Work out the finished part from the listing and answer in its coordinate system (mm). A direction names the side the tool comes from. Round coordinates to 2 decimals unless told otherwise and drop trailing zeros. Order: outer loops, then holes, each group sorted by start corner. A loop starts at its lowest first (then second) coordinate and runs counter-clockwise, first axis right, second up. Notation, with made-up numbers: (33.25, 48) - (79.25, 48) arc R17 ccw to (79.25, 53) - close; hole circle Ø2 at (50, -11.75). An arc over 180 degrees is marked (long way). Use one line per item in the form item = value. Start each with the question number.
Q1. For a pull along Y with two mould halves and no side action, classify faces 1 (the flat face through (-1, 10.514, -12)), 2 (the flat face through (40.64, 38, -20)), 3 (the cylindrical face through (39.388, 64.993, -18.568)) as +Y half, -Y half, draft (parallel to the pull), parting line (faces both ways), or undercut.
Q2. The part is cut by section C-C on y = 25.5. Determine the outline of the cut face in (x, z).
Q3. Which of the six approach directions +Z, -Z, +X, -X, +Y, -Y give full straight-line access (tool end or side, diameter ignored) to faces 4 (the flat face through (0, 62, -11)), 5 (the flat face through (19, 38, -25.4)), 6 (the flat face through (-1, 11.594, -1))?
Q4. The part is cut by section B-B on z = -11.43. State how many separate pieces and enclosed holes the cut face has, plus the area to 3 significant figures.
Q5. Given P1, Ø2.5, axis at y = 6.64, z = -16.38, coming from the -X side; P2, Ø3.5, axis at y = 67.16, z = -19.05, coming from the +X side; P3, Ø4, axis at x = 36, z = -18.5, coming from the +Y side, each flat-ended and moving along its own axis, determine where each tip first touches the part or whether it passes through.
Q6. Find the intervals of material crossed by line 1 (Y direction, x = 39.3, z = -19.05); line 2 (Z direction, x = 29.5, y = 38.5); line 3 (X direction, y = 53, z = -21.25), in increasing order. Write a range as [from, to].
from build123d import *

# Parameters (mm, degrees)
SKETCH1_W           = 43.18
SKETCH1_H           = 27.94
SKETCH1_W_2         = 38.1
SKETCH1_H_2         = 22.86
BOSS_EXTRUDE1_DEPTH = 76.2
CUT_EXTRUDE1_REACH  = 93.193
SKETCH3_R           = 2.2225
SKETCH3_R_2         = 6.99999997
CUT_EXTRUDE2_REACH  = 93.193
SKETCH2_W           = 19.91868
SKETCH2_H           = 38.1
SKETCH2_W_2         = 1.47066
SKETCH2_H_2         = 1.0795
SKETCH2_R           = 2.2225
FILLET1_R           = 1.27
FILLET2_R           = 1.27


# Some blends are built 0.0001 mm under size
with BuildPart() as part:
    # Sketch1 → Boss-Extrude1 (new body)
    with BuildSketch(Plane(origin=(0, 0, 0), x_dir=(1, 0, 0), z_dir=(0, 1, 0))):
        with Locations((19.05, 11.43)):
            Rectangle(SKETCH1_W, SKETCH1_H)
        with Locations((19.05, 11.43)):
            Rectangle(SKETCH1_W_2, SKETCH1_H_2, mode=Mode.SUBTRACT)
    extrude(amount=BOSS_EXTRUDE1_DEPTH)

    # Sketch3 → Cut-Extrude1 (cut, up to next)
    with BuildSketch(Plane(origin=(40.64, 0, 0), x_dir=(0, 0, -1), z_dir=(1, 0, 0)), mode=Mode.PRIVATE) as cut_extrude1_sk1:
        with Locations((19.05, 67.16268)):
            Circle(SKETCH3_R)
    cut_extrude1_tool1 = extrude(cut_extrude1_sk1.sketch, amount=-CUT_EXTRUDE1_REACH, mode=Mode.PRIVATE) & part.part
    # Sketch3 → Cut-Extrude1 (cut, up to next)
    with BuildSketch(Plane(origin=(40.64, 0, 0), x_dir=(0, 0, -1), z_dir=(1, 0, 0)), mode=Mode.PRIVATE) as cut_extrude1_sk2:
        with Locations((3.81, 67.16268)):
            Circle(SKETCH3_R)
    cut_extrude1_tool2 = extrude(cut_extrude1_sk2.sketch, amount=-CUT_EXTRUDE1_REACH, mode=Mode.PRIVATE) & part.part
    # Sketch3 → Cut-Extrude1 (cut, up to next)
    with BuildSketch(Plane(origin=(40.64, 0, 0), x_dir=(0, 0, -1), z_dir=(1, 0, 0)), mode=Mode.PRIVATE) as cut_extrude1_sk3:
        with Locations((19.05, 13.82268)):
            Circle(SKETCH3_R)
    cut_extrude1_tool3 = extrude(cut_extrude1_sk3.sketch, amount=-CUT_EXTRUDE1_REACH, mode=Mode.PRIVATE) & part.part
    # Sketch3 → Cut-Extrude1 (cut, up to next)
    with BuildSketch(Plane(origin=(40.64, 0, 0), x_dir=(0, 0, -1), z_dir=(1, 0, 0)), mode=Mode.PRIVATE) as cut_extrude1_sk4:
        with Locations((3.81, 13.82268)):
            Circle(SKETCH3_R)
    cut_extrude1_tool4 = extrude(cut_extrude1_sk4.sketch, amount=-CUT_EXTRUDE1_REACH, mode=Mode.PRIVATE) & part.part
    # Sketch3 → Cut-Extrude1 (cut, up to next)
    with BuildSketch(Plane(origin=(40.64, 0, 0), x_dir=(0, 0, -1), z_dir=(1, 0, 0)), mode=Mode.PRIVATE) as cut_extrude1_sk5:
        with Locations((11.43, 40.49268)):
            Circle(SKETCH3_R_2)
    cut_extrude1_tool5 = extrude(cut_extrude1_sk5.sketch, amount=-CUT_EXTRUDE1_REACH, mode=Mode.PRIVATE) & part.part
    add(cut_extrude1_tool1.solids().sort_by_distance((40.64, 67.16268, -19.05))[0], mode=Mode.SUBTRACT)
    add(cut_extrude1_tool2.solids().sort_by_distance((40.64, 67.16268, -3.81))[0], mode=Mode.SUBTRACT)
    add(cut_extrude1_tool3.solids().sort_by_distance((40.64, 13.82268, -19.05))[0], mode=Mode.SUBTRACT)
    add(cut_extrude1_tool4.solids().sort_by_distance((40.64, 13.82268, -3.81))[0], mode=Mode.SUBTRACT)
    add(cut_extrude1_tool5.solids().sort_by_distance((40.64, 40.49268, -11.43))[0], mode=Mode.SUBTRACT)

    # Sketch2 → Cut-Extrude2 (cut, up to next)
    with BuildSketch(Plane.ZY.offset(2.54), mode=Mode.PRIVATE) as cut_extrude2_sk1:
        with Locations((-11.43, 30.64383099)):
            Rectangle(SKETCH2_W, SKETCH2_H)
    cut_extrude2_tool1 = extrude(cut_extrude2_sk1.sketch, amount=-CUT_EXTRUDE2_REACH, mode=Mode.PRIVATE) & part.part
    # Sketch2 → Cut-Extrude2 (cut, up to next)
    with BuildSketch(Plane.ZY.offset(2.54), mode=Mode.PRIVATE) as cut_extrude2_sk2:
        with Locations((-22.12467, 30.64383099)):
            Rectangle(SKETCH2_W_2, SKETCH2_H)
    cut_extrude2_tool2 = extrude(cut_extrude2_sk2.sketch, amount=-CUT_EXTRUDE2_REACH, mode=Mode.PRIVATE) & part.part
    # Sketch2 → Cut-Extrude2 (cut, up to next)
    with BuildSketch(Plane.ZY.offset(2.54), mode=Mode.PRIVATE) as cut_extrude2_sk3:
        with Locations((-11.43, 50.23358099)):
            Rectangle(SKETCH2_W, SKETCH2_H_2)
    cut_extrude2_tool3 = extrude(cut_extrude2_sk3.sketch, amount=-CUT_EXTRUDE2_REACH, mode=Mode.PRIVATE) & part.part
    # Sketch2 → Cut-Extrude2 (cut, up to next)
    with BuildSketch(Plane.ZY.offset(2.54), mode=Mode.PRIVATE) as cut_extrude2_sk4:
        with Locations((-0.73533, 30.64383099)):
            Rectangle(SKETCH2_W_2, SKETCH2_H)
    cut_extrude2_tool4 = extrude(cut_extrude2_sk4.sketch, amount=-CUT_EXTRUDE2_REACH, mode=Mode.PRIVATE) & part.part
    # Sketch2 → Cut-Extrude2 (cut, up to next)
    with BuildSketch(Plane.ZY.offset(2.54), mode=Mode.PRIVATE) as cut_extrude2_sk5:
        with Locations((-11.43, 11.05408099)):
            Rectangle(SKETCH2_W, SKETCH2_H_2)
    cut_extrude2_tool5 = extrude(cut_extrude2_sk5.sketch, amount=-CUT_EXTRUDE2_REACH, mode=Mode.PRIVATE) & part.part
    # Sketch2 → Cut-Extrude2 (cut, up to next)
    with BuildSketch(Plane.ZY.offset(2.54), mode=Mode.PRIVATE) as cut_extrude2_sk6:
        with Locations((-6.47954, 6.64337099)):
            Circle(SKETCH2_R)
    cut_extrude2_tool6 = extrude(cut_extrude2_sk6.sketch, amount=-CUT_EXTRUDE2_REACH, mode=Mode.PRIVATE) & part.part
    # Sketch2 → Cut-Extrude2 (cut, up to next)
    with BuildSketch(Plane.ZY.offset(2.54), mode=Mode.PRIVATE) as cut_extrude2_sk7:
        with Locations((-16.38046, 6.64337099)):
            Circle(SKETCH2_R)
    cut_extrude2_tool7 = extrude(cut_extrude2_sk7.sketch, amount=-CUT_EXTRUDE2_REACH, mode=Mode.PRIVATE) & part.part
    # Sketch2 → Cut-Extrude2 (cut, up to next)
    with BuildSketch(Plane.ZY.offset(2.54), mode=Mode.PRIVATE) as cut_extrude2_sk8:
        with Locations((-16.38046, 54.64429099)):
            Circle(SKETCH2_R)
    cut_extrude2_tool8 = extrude(cut_extrude2_sk8.sketch, amount=-CUT_EXTRUDE2_REACH, mode=Mode.PRIVATE) & part.part
    # Sketch2 → Cut-Extrude2 (cut, up to next)
    with BuildSketch(Plane.ZY.offset(2.54), mode=Mode.PRIVATE) as cut_extrude2_sk9:
        with Locations((-6.47954, 54.64429099)):
            Circle(SKETCH2_R)
    cut_extrude2_tool9 = extrude(cut_extrude2_sk9.sketch, amount=-CUT_EXTRUDE2_REACH, mode=Mode.PRIVATE) & part.part
    add(cut_extrude2_tool1.solids().sort_by_distance((-2.54, 30.643831, -11.43))[0], mode=Mode.SUBTRACT)
    add(cut_extrude2_tool2.solids().sort_by_distance((-2.54, 30.643831, -22.12467))[0], mode=Mode.SUBTRACT)
    add(cut_extrude2_tool3.solids().sort_by_distance((-2.54, 50.233581, -11.43))[0], mode=Mode.SUBTRACT)
    add(cut_extrude2_tool4.solids().sort_by_distance((-2.54, 30.643831, -0.73533))[0], mode=Mode.SUBTRACT)
    add(cut_extrude2_tool5.solids().sort_by_distance((-2.54, 11.054081, -11.43))[0], mode=Mode.SUBTRACT)
    add(cut_extrude2_tool6.solids().sort_by_distance((-2.54, 6.643371, -6.47954))[0], mode=Mode.SUBTRACT)
    add(cut_extrude2_tool7.solids().sort_by_distance((-2.54, 6.643371, -16.38046))[0], mode=Mode.SUBTRACT)
    add(cut_extrude2_tool8.solids().sort_by_distance((-2.54, 54.644291, -16.38046))[0], mode=Mode.SUBTRACT)
    add(cut_extrude2_tool9.solids().sort_by_distance((-2.54, 54.644291, -6.47954))[0], mode=Mode.SUBTRACT)

    # Fillet1
    # the kernel refuses this fillet: 1.27 mm, written as the material it adds along each edge
    with BuildSketch(Plane(origin=(-2.54, 10.51433099, -1.47066), x_dir=(0, 0, -1), z_dir=(1, 0, 0)), Plane(origin=(-2.54, 50.77333099, -21.38934), x_dir=(0, 0, 1), z_dir=(1, 0, 0))) as fillet1_piece_1:
        with BuildLine():
            CenterArc((1.255631216, 1.27), FILLET1_R, 188.626926559, 81.373073441)
            Line((0, 1.0795), (-0.025112624, 1.07569))
            ThreePointArc((-0.025112624, 1.07569), (-0.0254, 0.53975), (-0.0254, 0))
            Line((-0.0254, 0), (0, -0.0254))
            Line((0, -0.0254), (1.255631216, -0.0254))
            Line((1.255631216, -0.0254), (1.255631216, 0))
        make_face()
    extrude(amount=2.54)
    with BuildSketch(Plane(origin=(-2.54, 10.51433099, -21.38934), x_dir=(0, 1, 0), z_dir=(1, 0, 0)), Plane(origin=(-2.54, 50.77333099, -1.47066), x_dir=(0, -1, 0), z_dir=(1, 0, 0))) as fillet1_piece_2:
        with BuildLine():
            CenterArc((1.27, 1.255631216), FILLET1_R, 180, 81.373073441)
            Line((0, 1.255631216), (-0.0254, 1.255631216))
            Line((-0.0254, 1.255631216), (-0.0254, 0))
            Line((-0.0254, 0), (0, -0.0254))
            ThreePointArc((0, -0.0254), (0.53975, -0.0254), (1.07569, -0.025112624))
            Line((1.07569, -0.025112624), (1.0795, 0))
        make_face()
    extrude(amount=2.54)

    # Fillet2
    fillet2_edges = [part.edges().sort_by_distance(p)[0] for p in [
        (40.64, 76.2, -11.43),
        (0, 0, -11.43),
        (0, 62.946915495, -22.86),
        (19.05, 0, 0),
        (0, 62.946915495, 0),
        (38.1, 0, -11.43),
        (38.1, 38.1, 0),
        (19.05, 0, -22.86),
        (38.1, 38.1, -22.86),
        (0, 76.2, -11.43),
        (19.05, 76.2, -25.4),
        (19.05, 76.2, 0),
        (38.1, 76.2, -11.43),
        (19.05, 76.2, -22.86),
        (-2.54, 76.2, -11.43),
        (19.05, 0, -25.4),
        (0, 5.796915495, -22.86),
        (0, 5.796915495, 0),
        (40.64, 0, -11.43),
        (19.05, 0, 2.54),
        (-2.54, 0, -11.43),
        (-2.54, 38.1, -25.4),
        (40.64, 38.1, -25.4),
        (40.64, 38.1, 2.54),
        (-2.54, 38.1, 2.54),
        (19.05, 76.2, 2.54),
    ]]
    fillet(fillet2_edges, radius=FILLET2_R - 0.0001)  # a hair under: the kernel refuses the full size


solid = part.part
Found:
q1.face_1 = undercut
q1.face_2 = draft
q1.face_3 = undercut
q2.outline = (-2.54, -24.13) arc R1.27 ccw to (-1.27, -25.4) - (39.37, -25.4) arc R1.27 ccw to (40.64, -24.13) - (40.64, 1.27) arc R1.27 ccw to (39.37, 2.54) - (-1.27, 2.54) arc R1.27 ccw to (-2.54, 1.27) - (-2.54, 0) - (36.83, 0) arc R1.27 cw to (38.1, -1.27) - (38.1, -21.59) arc R1.27 cw to (36.83, -22.86) - (-2.54, -22.86) - close
q3.face_4 = +Y, -Y
q3.face_5 = -Z, +X, -X, +Y, -Y
q3.face_6 = -X
q4.separate_pieces = 4
q4.enclosed_holes = 0
q4.area = 247 mm²
q5.P1 = 38.1
q5.P2 = 0
q5.P3 = through
q6.line_1 = [0, 11.6], [16.05, 64.94], [69.39, 76.2]
q6.line_2 = [-25.4, -22.86], [0, 2.54]
q6.line_3 = [-2.54, 0], [38.1, 40.64]
